```python
from build123d import *
from OCP.BRepFilletAPI import BRepFilletAPI_MakeChamfer

# Parameters (mm, degrees)
SKETCH1_R           = 12.7
BOSS_EXTRUDE1_DEPTH = 31.1658
SKETCH2_R           = 12.7
SKETCH2_R_2         = 3.2385
CUT_EXTRUDE1_DEPTH  = 12.7
CUT_EXTRUDE2_START  = -8.89
SKETCH3_R           = 12.7
SKETCH3_R_2         = 7.14375
CUT_EXTRUDE2_DEPTH  = 8.89
CHAMFER1_SIZE       = 1.27
SKETCH4_R           = 12.7
SKETCH4_R_2         = 7.747
BOSS_EXTRUDE2_DEPTH = 15.24
CHAMFER2_SIZE       = 2.54
SKETCH6_R           = 1.5875
SKETCH6_R_2         = 1.651
CUT_EXTRUDE3_DEPTH  = 50.8
SKETCH7_R           = 14.605
SKETCH7_R_2         = 10.795
BOSS_EXTRUDE3_DEPTH = 19.05
CHAMFER3_SIZE       = 1.27
CHAMFER3_SIZE2      = 2.54


with BuildPart() as part:
    # Sketch1 → Boss-Extrude1 (new body)
    with BuildSketch(Plane(origin=(0, 0, 0), x_dir=(1, 0, 0), z_dir=(0, 1, 0))):
        with Locations(Location((0, 0, 0), (0, 0, 270))):
            Circle(SKETCH1_R)
    extrude(amount=BOSS_EXTRUDE1_DEPTH)

    # Sketch2 → Cut-Extrude1 (cut)
    with BuildSketch(Plane.XZ):
        with Locations(Location((0, 0, 0), (0, 0, 270))):
            Circle(SKETCH2_R)
        with Locations(Location((0, 0, 0), (0, 0, 270))):
            Circle(SKETCH2_R_2, mode=Mode.SUBTRACT)
    extrude(amount=-CUT_EXTRUDE1_DEPTH, mode=Mode.SUBTRACT)

    # Sketch3 → Cut-Extrude2 (cut)
    with BuildSketch(Plane(origin=(0, 31.1658, 0), x_dir=(1, 0, 0), z_dir=(0, 1, 0)).offset(CUT_EXTRUDE2_START)):
        with Locations(Location((0, 0, 0), (0, 0, 90))):
            Circle(SKETCH3_R)
        with Locations(Location((0, 0, 0), (0, 0, 270))):
            Circle(SKETCH3_R_2, mode=Mode.SUBTRACT)
    extrude(amount=CUT_EXTRUDE2_DEPTH, mode=Mode.SUBTRACT)

    # Chamfer1
    chamfer1_edges = [part.edges().sort_by_distance(p)[0] for p in [
        (0, 31.1658, -7.14375),
        (0, 0, 3.2385),
    ]]
    chamfer(chamfer1_edges, length=CHAMFER1_SIZE)

    # Sketch4 → Boss-Extrude2 (add)
    with BuildSketch(Plane.XZ):
        with Locations(Location((0, 0, 0), (0, 0, 270))):
            Circle(SKETCH4_R)
        with Locations(Location((0, 0, 0), (0, 0, 270))):
            Circle(SKETCH4_R_2, mode=Mode.SUBTRACT)
    extrude(amount=-BOSS_EXTRUDE2_DEPTH)

    # Chamfer2
    chamfer2_edges = [part.edges().sort_by_distance(p)[0] for p in [
        (0, 0, 7.747),
    ]]
    chamfer(chamfer2_edges, length=CHAMFER2_SIZE)

    # Sketch6 → Cut-Extrude3 (cut, symmetric)
    with BuildSketch(Plane.XY):
        with Locations((0, 6.35)):
            Circle(SKETCH6_R)
        with Locations((0, 26.0858)):
            Circle(SKETCH6_R_2)
    extrude(amount=CUT_EXTRUDE3_DEPTH, both=True, mode=Mode.SUBTRACT)

    # Sketch7 → Boss-Extrude3 (add)
    with BuildSketch(Plane.XZ):
        with Locations(Location((0, 0, 0), (0, 0, 90))):
            Circle(SKETCH7_R)
        with Locations(Location((0, 0, 0), (0, 0, 90))):
            Circle(SKETCH7_R_2, mode=Mode.SUBTRACT)
    extrude(amount=BOSS_EXTRUDE3_DEPTH)

    # Chamfer3: one chamfer whose edges measure the first distance from different faces: ONE call of the kernel's chamfer builder (chamfer() names one face for all edges)
    chamfer3_edges_1 = [part.edges().sort_by_distance(p)[0] for p in [
        (0, 0, -14.605),
    ]]
    chamfer3_side_1 = [part.faces().sort_by_distance(p)[0] for p in [
        (0, 0, -14.191908218),
    ]]
    chamfer3_edges_2 = [part.edges().sort_by_distance(p)[0] for p in [
        (0, -19.05, -10.795),
    ]]
    chamfer3_side_2 = [part.faces().sort_by_distance(p)[0] for p in [
        (0, -19.05, -14.191908218),
    ]]
    chamfer3 = BRepFilletAPI_MakeChamfer(part.part.solid().wrapped)
    for e in chamfer3_edges_1:
        chamfer3.Add(CHAMFER3_SIZE, CHAMFER3_SIZE2, e.wrapped, chamfer3_side_1[0].wrapped)  # the first distance lies on this face
    for e in chamfer3_edges_2:
        chamfer3.Add(CHAMFER3_SIZE, CHAMFER3_SIZE2, e.wrapped, chamfer3_side_2[0].wrapped)  # the first distance lies on this face
    add(Compound.cast(chamfer3.Shape()), mode=Mode.REPLACE)


solid = part.part
```
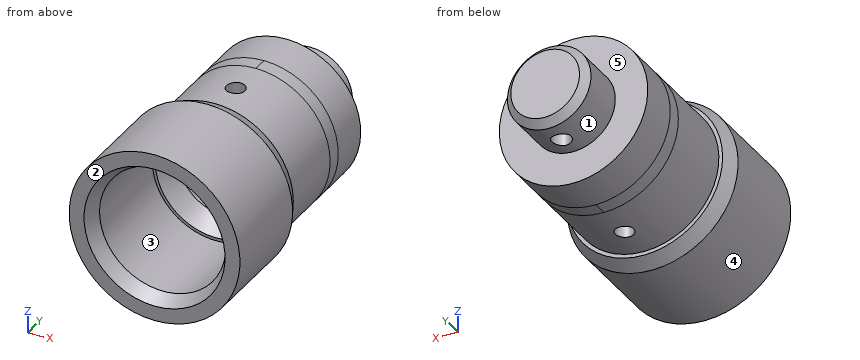
Model file for the job. Use its own axes, mm. Face numbers are marked on the shaded views. A direction names the side the tool comes from. Coordinates: 2 decimals unless noted, no trailing zeros. Write each loop counter-clockwise with the first axis right and the second up, starting at its lowest first coordinate (ties: lowest second). Pieces come first, ordered by that corner, then holes. Notation, with made-up numbers: (12, 56) - (49, 56) arc R18 ccw to (49, 65) - close; hole circle Ø9 at (-13.75, 1.25). An arc over 180 degrees is marked (long way). Use a Markdown table: item, result. Add a question column.
Item 1: Band-saw the part on C-C, the plane x = 1. Give the number of separate pieces and of enclosed holes in the cut face, and give its area (3 significant figures).
Item 2: Band-saw the part on B-B, the plane y = 16. Write the cut outline in (x, z).
Item 3: Two-plate mould, pull along X, no slides. Class the marked faces 3, 4 and 5: pulls with the +X half, pulls with the -X half, needs draft (parallel to the pull), parting line crosses it, or undercut.
Item 4: Band-saw the part on A-A, the plane y = 6.35. Write the cut outline in (x, z).
Item 5: 3-axis set-ups, long thin cutter, end or side, ignore diameter. For the marked faces 1 and 2: which of +Z, -Z, +X, -X, +Y, -Y reach the whole face in a straight line?
Item 6: Drop flat-ended pins along their axis: pin 1 (3 mm diameter, centred on y = -5.5, z = 1, fed in from -X) (3 decimals); pin 2 (10 mm diameter, centred on y = -3, z = 11, fed in from -X); pin 3 (1.5 mm diameter, centred on x = 1.5, y = 21, fed in from +Z); pin 4 (5 mm diameter, centred on x = 0, y = 6.35, fed in from -Z). Give the stop position or say it passes through.
Item 7: Drill centre lines: line 1 along Z through (x, y) = (0, 10); line 2 along X through (y, z) = (6.35, 2.2). Where is each one in solid material? Low to high.
Item 8: Band-saw the part on D-D, the plane y = -15. Write the cut outline in (x, z) (3 decimals).
A:
| question | item | result |
|---|---|---|
| 1 | separate pieces | 5 |
| 1 | enclosed holes | 0 |
| 1 | area | 625 mm² |
| 2 | outline | circle Ø25.4 at (0, 0) |
| 3 | face 3 | undercut |
| 3 | face 4 | parting line crosses it |
| 3 | face 5 | needs draft |
| 4 | outline | (-1.59, -12.6) - (-1.59, -7.58) arc R7.75 cw to (-1.59, 7.58) - (-1.59, 12.6) arc R12.7 ccw to start; (-1.59, -2.82) - (-1.59, 2.82) arc R3.24 ccw to start; (1.59, -12.6) arc R12.7 ccw to (1.59, 12.6) - (1.59, 7.58) arc R7.75 cw to (1.59, -7.58) - close; (1.59, -2.82) arc R3.24 ccw to (1.59, 2.82) - close |
| 5 | face 1 | +Y |
| 5 | face 2 | +Z, -Z, +X, -X, -Y |
| 6 | pin 1 | stops at x = -14.605 |
| 6 | pin 2 | stops at x = -13.32 |
| 6 | pin 3 | stops at z = 12.68 |
| 6 | pin 4 | stops at z = -12.7 |
| 7 | line 1 | z = -12.7 to -7.75, -3.24 to 3.24, 7.75 to 12.7 |
| 7 | line 2 | x = -12.51 to -7.43, -2.38 to -1.59, 1.59 to 2.38, 7.43 to 12.51 |
| 8 | outline | circle Ø29.21 at (0, 0); hole circle Ø21.59 at (0, 0) |
